```python
from build123d import *

# Parameters (mm, degrees)
SKETCH1_R                    = 152.4
BOSS_EXTRUDE1_DEPTH          = 20
F_3_8_0_375_DIAMETER_HOLE1_D = 9.525
CIRPATTERN1_COUNT            = 8
SKETCH5_R                    = 55
CUT_EXTRUDE1_DEPTH           = 217.452119417


with BuildPart() as part:
    # Sketch1 → Boss-Extrude1 (new body)
    with BuildSketch(Plane.XY):
        Circle(SKETCH1_R)
    extrude(amount=BOSS_EXTRUDE1_DEPTH)

    # 3/8 (0.375) Diameter Hole1 (through all)
    with Locations(Plane(origin=(0, 0, 0), x_dir=(-1, 0, 0), z_dir=(0, 0, -1))):
        with Locations((-65.2, 0)):
            f_3_8_0_375_diameter_hole1 = Hole(F_3_8_0_375_DIAMETER_HOLE1_D / 2)

    # CirPattern1: 3/8 (0.375) Diameter Hole1 ×8 about axis
    cirpattern1_axis = Axis((-0.063734115, 0, 0), (0, 0, 1))
    for i in range(1, CIRPATTERN1_COUNT):
        add(f_3_8_0_375_diameter_hole1.rotate(cirpattern1_axis, i * 360 / CIRPATTERN1_COUNT), mode=Mode.SUBTRACT)

    # Sketch5 → Cut-Extrude1 (cut, through all)
    with BuildSketch(Plane(origin=(0, 0, 0), x_dir=(-1, 0, 0), z_dir=(0, 0, -1))):
        Circle(SKETCH5_R)
    extrude(amount=-CUT_EXTRUDE1_DEPTH, mode=Mode.SUBTRACT)


solid = part.part
```
Geometry check sheet. Reference: the model listing, model coordinates, mm. Give positions to 0.01 mm unless a question says otherwise; leave off trailing zeros. Order: outer loops, then holes, each group sorted by start corner. A loop starts at its lowest first (then second) coordinate and runs counter-clockwise, first axis right, second up. Notation, with made-up numbers: (-13, 50.5) -> (42, 50.5) arc R26 ccw to (42, 81.5) -> close; hole circle Ø9 at (75, -25.5). An arc over 180 degrees is marked (long way). Write each question's results on one line, items separated by ' | '. Start each with the question number.
(1) Sectioned sample at D-D (x = -37). Enter the section's corners in (y, z), plus the area to 3 significant figures.
(2) Sectioned sample at C-C (z = 9.5). Give the number of separate pieces and of enclosed holes in the cut face, plus the area to 3 significant figures.
(3) Scan lines: line 1 (Y direction, x = 3.5, z = 13.25); line 2 (X direction, y = 2, z = 6.75); line 3 (Y direction, x = -8, z = 6.25). Record each from-to range of solid material in increasing order.
(4) Mould release check, pull along X, two halves, no side actions. Record for faces 1 (the face through (-41.454, -45.942, 10.14)), 2 (the face through (66, -32, 20)), 3 (the face through (-120.94, -92.73, 9.86)): pulls with the +X half, pulls with the -X half, needs draft (parallel to the pull), parting line crosses it, or undercut.
(5) Sectioned sample at A-A (y = 0). Enter the section's corners in (x, z).
(6) Gauge pin test, flat ends, axial feed: P1, Ø8.5, axis at x = -0.06, y = 65.26, coming from the +Z side; P2, Ø2, axis at x = 114.5, z = 10.5, coming from the -Y side; P3, Ø12.5, axis at x = 46.08, y = 46.15, coming from the +Z side; P4, Ø4, axis at y = -91, z = 2, coming from the -X side. Record the tip position at first contact, or that the pin passes through.
(7) Sectioned sample at B-B (x = 26.5). Enter the section's corners in (y, z), plus the area to 3 significant figures.
Answer below:
1) outline: (-147.84, 0) -> (-40.69, 0) -> (-40.69, 20) -> (-147.84, 20) -> close; (40.69, 0) -> (147.84, 0) -> (147.84, 20) -> (40.69, 20) -> close | area: 4,290 mm2
2) separate pieces: 1 | enclosed holes: 9 | area: 62,900 mm2
3) line 1: -152.36 to -68.42, -62.1 to -54.89, 54.89 to 62.1, 68.42 to 152.36 | line 2: -152.39 to -69.65, -61.01 to -54.96, 54.96 to 60.88, 69.52 to 152.39 | line 3: -152.19 to -54.42, 54.42 to 152.19
4) face 1: undercut | face 2: needs draft | face 3: parting line crosses it
5) outline: (-152.4, 0) -> (-70.09, 0) -> (-70.09, 20) -> (-152.4, 20) -> close; (-60.56, 0) -> (-55, 0) -> (-55, 20) -> (-60.56, 20) -> close; (55, 0) -> (60.44, 0) -> (60.44, 20) -> (55, 20) -> close; (69.96, 0) -> (152.4, 0) -> (152.4, 20) -> (69.96, 20) -> close
6) P1: through | P2: y = -101.7 | P3: z = 20 | P4: x = -123.71
7) outline: (-150.08, 0) -> (-48.19, 0) -> (-48.19, 20) -> (-150.08, 20) -> close; (48.19, 0) -> (150.08, 0) -> (150.08, 20) -> (48.19, 20) -> close | area: 4,080 mm2
